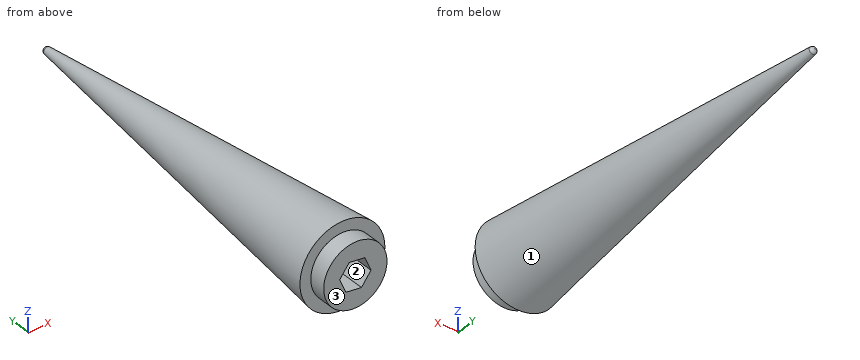
Autodesk Fusion 360 part; units mm, degrees
sketch "base" plane through (0, 0, 0) normal (0, 1, 0) x (1, 0, 0)
  circle A0 centre (0, 0) radius 12.75
  circle A1 centre (0, 0) radius 9.5
  line L0 (4.6976, 0.5881) -> (1.8395, 4.3623)
  line L1 (1.8395, 4.3623) -> (-2.8581, 3.7742)
  line L2 (-2.8581, 3.7742) -> (-4.6976, -0.5881)
  line L3 (-4.6976, -0.5881) -> (-1.8395, -4.3623)
  line L4 (-1.8395, -4.3623) -> (2.8581, -3.7742)
  line L5 (2.8581, -3.7742) -> (4.6976, 0.5881)
  dimension "d1" = 25.5
  dimension "d8" = 19
  dimension "d11" = 4.1
sketch "side" plane through (0, 0, 0) normal (0, 0, 1) x (1, 0, 0)
  line L0 (0, 0) -> (0, 115)
  line L1 (0, 0) -> (12.75, 0)
  line L2 (0, 115) -> (1, 115)
  line L3 (1, 115) -> (12.75, 0)
  line L4 (0, 108.2663) -> (1.688, 108.2663)
  dimension "d4" = 115
  dimension "d5" = 12.75
  dimension "d19" = 1
revolve "cone" add sketch "side" angle 360 about axis through (0, 0, 0) along (0, 1, 0) makes body 1
extrude "tip_insert" cut sketch "base" along normal blind 5 contours A1 | L0 L1 L2 L3 L4 L5 bodies 1
extrude "shoulder" add sketch "base" along normal blind 10 and the other way blind 5 separate body contours A1 | L0 L1 L2 L3 L4 L5 makes body 2
extrude "Extrude2" cut sketch "base" along normal blind 25 from surface at -5 contours L0 L1 L2 L3 L4 L5 bodies 2
fillet "Fillet1" radius 1 1 edges at (-0.9323, 115, -0.3616) on bodies 1
combine "Combine1" operation add target body 1 tool bodies 2
equation "d1 = base_diam"
equation "base_diam = 25.5 mm"
equation "height = 115 mm"
equation "d4 = height"
equation "d5 = base_diam / 2"
equation "inside_diam = 19 mm"
equation "d8 = inside_diam"
Could you check a few things on this model? Use its own coordinates, in mm. Face numbers are marked on the shaded views. Give positions to 0.01 mm unless a question says otherwise; leave off trailing zeros. Order: outer loops, then holes, each group sorted by start corner. A loop starts at its lowest first (then second) coordinate and runs counter-clockwise, first axis right, second up. Notation, with made-up numbers: (-32.5, -33.5) - (11.5, -33.5) arc R14 ccw to (11.5, -23.5) - close; hole circle Ø9 at (26.5, -36.5). An arc over 180 degrees is marked (long way). One line per item, written item: value. Start each with the question number.
1. For P1, Ø5, axis at x = 7, y = 9.5, coming from the -Z side; P2, Ø1.5, axis at x = -0.5, y = 32.5, coming from the +Z side; P3, Ø12, axis at y = 59, z = 0, coming from the -X side; P4, Ø8, axis at x = -9, z = -4.5, coming from the -Y side, each with a flat end and sliding along its axis, tell me the tip position at first contact or that it passes through.
2. Imagine slicing it at B-B on y = 47. List the corners of the cut face in (x, z) for me.
3. Imagine slicing it at A-A on y = 22.5. List the corners of the cut face in (x, z) for me.
4. Thinking about a two-plate mould opening in X: for the marked faces 1, 2 and 3, which applies, +X half, -X half, draft (parallel to the pull), parting line (faces both ways), or undercut?
5. If I drill on probe 1 along X at (y, z) = (46, 1.25); probe 2 along Z at (x, y) = (0.5, 57.5); probe 3 along X at (y, z) = (90.5, -2.5), over which ranges is the centre line in solid material (lowest first)?
Values:
1. P1: z = -10.92
1. P2: z = 9.5
1. P3: x = -7.33
1. P4: y = -5
2. outline: circle Ø15.9 at (0, 0)
3. outline: circle Ø20.9 at (0, 0)
4. face 1: parting line
4. face 2: undercut
4. face 3: draft
5. probe 1: -7.95 to 7.95
5. probe 2: -6.86 to 6.86
5. probe 3: -2.45 to 2.45
